Read the model definition and answer for the solid it produces. Units are mm, in the model's axes. Coordinates: 2 decimals unless noted, no trailing zeros. Order: outer loops, then holes, each group sorted by start corner. A loop starts at its lowest first (then second) coordinate and runs counter-clockwise, first axis right, second up. Notation, with made-up numbers: M 60.25,27 L 87.25,27 A21 ccw 87.25,34 Z; hole C -7,-39 d10. An arc over 180 degrees is marked long. Use a Markdown table: item, result. Add a question column.
1) Find section A-A on x = 0. Write down the section's boundary in (y, z).
2) Each of these flat-tipped pins is pushed along its axis until it touches: pin 1 Ø5 at (x, y) = (-6.5, 20) entering from +Z; pin 2 Ø8 at (y, z) = (8.5, 60.5) entering from +X; pin 3 Ø12 at (x, z) = (-55, 56) entering from +Y; pin 4 Ø4 at (y, z) = (12.7, -12.7) entering from -X. Where does it stop, or does it pass through?
3) Find section D-D on y = 12.7. Count the separate pieces of the cut face and the enclosed holes in it, plus the area to 3 significant figures.
4) The mould has two halves that part along Y. Classify faces 1 (the face through (76, 25.4, -12)), 2 (the face through (59.02, 12.98, -50.05)), 3 (the face through (76, 0, -12)): released by +Y, released by -Y, zero draft, split by the parting line, or undercut.
5) Find section B-B on z = 0. Write down the section's boundary in (x, y).
6) Find the intervals of material crossed by probe 1 along Z at (x, y) = (4.5, 22); probe 2 along Y at (x, z) = (76.8, -12.7); probe 3 along X at (y, z) = (14.5, -17), in increasing order. Write a range as [from, to].
7) Find section C-C on z = -47. Write down the section's boundary in (x, y).
from build123d import *

# Parameters (mm, degrees)
SKETCH1_R                                    = 78.359
SKETCH1_R_2                                  = 76.1746
BOSS_EXTRUDE1_DEPTH                          = 25.4
SKETCH2_R                                    = 2.18313
SKETCH2_W                                    = 9.906
SKETCH2_H                                    = 9.906
CUT_EXTRUDE1_DEPTH                           = 114.690042493
MIRROR2_AT_THE_SECOND_PLANE_COPY_1_SKETC_R   = 78.359
MIRROR2_AT_THE_SECOND_PLANE_COPY_1_SKETC_R_2 = 76.1746
MIRROR2_AT_THE_SECOND_PLANE_COPY_1_DEPTH     = 25.4
MIRROR2_AT_THE_SECOND_PLANE_COPY_2_SKETC_R   = 2.18313
MIRROR2_AT_THE_SECOND_PLANE_COPY_2_SKETC_W   = 9.906
MIRROR2_AT_THE_SECOND_PLANE_COPY_2_SKETC_H   = 9.906
MIRROR2_AT_THE_SECOND_PLANE_COPY_2_DEPTH     = 114.690042493
SKETCH3_R                                    = 6.35
CUT_EXTRUDE2_DEPTH                           = 114.690042653
CUT_EXTRUDE2_DEPTH_BACK                      = 114.690042653


with BuildPart() as part:
    # Sketch1 → Boss-Extrude1 (new body)
    with BuildSketch(Plane(origin=(0, 0, 0), x_dir=(1, 0, 0), z_dir=(0, 1, 0))):
        with Locations(Location((0, 0, 0), (0, 0, 270))):
            Circle(SKETCH1_R)
        with Locations(Location((0, 0, 0), (0, 0, 270))):
            Circle(SKETCH1_R_2, mode=Mode.SUBTRACT)
    boss_extrude1 = extrude(amount=BOSS_EXTRUDE1_DEPTH)

    # Sketch2 → Cut-Extrude1 (cut, symmetric)
    with BuildSketch(Plane(origin=(0, 0, 0), x_dir=(0, 0, -1), z_dir=(1, 0, 0))):
        with Locations(Location((-12.7, 12.7, 0), (0, 0, 180))):
            Circle(SKETCH2_R)
        with Locations(Location((12.7, 12.7, 0), (0, 0, 180))):
            Circle(SKETCH2_R)
        with Locations((0, 12.7)):
            Rectangle(SKETCH2_W, SKETCH2_H)
    cut_extrude1 = extrude(amount=CUT_EXTRUDE1_DEPTH, both=True, mode=Mode.SUBTRACT)



with BuildPart() as mirror2_1:
    # Mirror2: Boss-Extrude1 across plane
    add(boss_extrude1.mirror(Plane(origin=(0, 0, 0), x_dir=(0, 0, 1), z_dir=(1, 0, 0))))

    # Mirror2 2: Cut-Extrude1 across plane
    add(cut_extrude1.mirror(Plane(origin=(0, 0, 0), x_dir=(0, 0, 1), z_dir=(1, 0, 0))), mode=Mode.SUBTRACT)


with BuildPart() as part_1:
    add(part.part)

    add(mirror2_1.part)  # Mirror2 at the second plane merges Mirror2_1
    # Mirror2 at the second plane: Boss-Extrude1, Cut-Extrude1 across plane
    add(boss_extrude1.mirror(Plane.ZX.offset(12.7)))
    add(cut_extrude1.mirror(Plane.ZX.offset(12.7)), mode=Mode.SUBTRACT)

    # Mirror2 at the second plane copy 1 sketc → Mirror2 at the second plane copy 1 (add)
    with BuildSketch(Plane(origin=(0, 25.4, 0), x_dir=(-1, 0, 0), z_dir=(0, -1, 0))):
        with Locations(Location((0, 0, 0), (0, 0, 270))):
            Circle(MIRROR2_AT_THE_SECOND_PLANE_COPY_1_SKETC_R)
        with Locations(Location((0, 0, 0), (0, 0, 270))):
            Circle(MIRROR2_AT_THE_SECOND_PLANE_COPY_1_SKETC_R_2, mode=Mode.SUBTRACT)
    extrude(amount=MIRROR2_AT_THE_SECOND_PLANE_COPY_1_DEPTH)

    # Mirror2 at the second plane copy 2 sketc → Mirror2 at the second plane copy 2 (cut, symmetric)
    with BuildSketch(Plane(origin=(0, 25.4, 0), x_dir=(0, 0, -1), z_dir=(-1, 0, 0))):
        with Locations(Location((-12.7, 12.7, 0), (0, 0, 180))):
            Circle(MIRROR2_AT_THE_SECOND_PLANE_COPY_2_SKETC_R)
        with Locations(Location((12.7, 12.7, 0), (0, 0, 180))):
            Circle(MIRROR2_AT_THE_SECOND_PLANE_COPY_2_SKETC_R)
        with Locations((0, 12.7)):
            Rectangle(MIRROR2_AT_THE_SECOND_PLANE_COPY_2_SKETC_W, MIRROR2_AT_THE_SECOND_PLANE_COPY_2_SKETC_H)
    extrude(amount=MIRROR2_AT_THE_SECOND_PLANE_COPY_2_DEPTH, both=True, mode=Mode.SUBTRACT)

    # Sketch3 → Cut-Extrude2 (cut, two sides)
    with BuildSketch(Plane(origin=(0, 0, 0), x_dir=(-0.7071067811865477, 0, -0.7071067811865475), z_dir=(0.7071067811865475, 0, -0.7071067811865477))) as cut_extrude2_sk:
        with Locations((0, 12.7)):
            Circle(SKETCH3_R)
    extrude(amount=CUT_EXTRUDE2_DEPTH, mode=Mode.SUBTRACT)
    extrude(cut_extrude2_sk.sketch, amount=-CUT_EXTRUDE2_DEPTH_BACK, mode=Mode.SUBTRACT)


solid = part_1.part
Check result:
| question | item | result |
|---|---|---|
| 1 | outline | M 0,-78.36 L 25.4,-78.36 L 25.4,-76.17 L 0,-76.17 Z; M 0,76.17 L 25.4,76.17 L 25.4,78.36 L 0,78.36 Z |
| 2 | pin 1 | stops at z = 78.26 |
| 2 | pin 2 | stops at x = 54.29 |
| 2 | pin 3 | stops at y = 25.4 |
| 2 | pin 4 | passes through |
| 3 | separate pieces | 8 |
| 3 | enclosed holes | 0 |
| 3 | area | 923 mm2 |
| 4 | face 1 | released by +Y |
| 4 | face 2 | undercut |
| 4 | face 3 | released by -Y |
| 5 | outline | M -78.36,0 L -76.17,0 L -76.17,7.75 L -78.36,7.75 Z; M -78.36,17.65 L -76.17,17.65 L -76.17,25.4 L -78.36,25.4 Z; M 76.17,0 L 78.36,0 L 78.36,7.75 L 76.17,7.75 Z; M 76.17,17.65 L 78.36,17.65 L 78.36,25.4 L 76.17,25.4 Z |
| 6 | probe 1 | z = [-78.23, -76.04], [76.04, 78.23] |
| 6 | probe 2 | y = [0, 10.52], [14.88, 25.4] |
| 6 | probe 3 | x = [-76.49, -74.25], [74.25, 76.49] |
| 7 | outline | M -62.7,0 L -59.95,0 L -59.95,25.4 L -62.7,25.4 Z; M 59.95,0 L 62.7,0 L 62.7,25.4 L 59.95,25.4 Z |
